from build123d import *

# Parameters (mm, degrees)
F1_DEPTH       = 16
F3_D           = 3.15
F3_CBORE_D     = 6.5
F3_CBORE_DEPTH = 3


with BuildPart() as f1:
    # F0 (on Top) → F1 (new body, symmetric)
    with BuildSketch(Plane.XY):
        with BuildLine():
            Line((4, 3), (-4, 3))
            ThreePointArc((-4, 3), (0, -5), (4, 3))
        make_face()
    extrude(amount=F1_DEPTH, both=True)

    # F3 (through all)
    with Locations(Plane(origin=(0, 3, 0), x_dir=(-1, 0, 0), z_dir=(0, 1, 0))):
        with Locations((0, 8), (0, -8)):
            CounterBoreHole(F3_D / 2, F3_CBORE_D / 2, F3_CBORE_DEPTH)


solid = f1.part
Can you work these out from the model? Positions are in its coordinate system, mm. A direction names the side the tool comes from. Coordinates: 2 decimals unless noted, no trailing zeros. Write each loop counter-clockwise with the first axis right and the second up, starting at its lowest first coordinate (ties: lowest second). Pieces come first, ordered by that corner, then holes. Notation, with made-up numbers: (41.25, 50.5) -> (72.25, 50.5) arc R22 cw to (72.25, 81.5) -> close; hole circle Ø9 at (66.5, 12). An arc over 180 degrees is marked (long way). Write item = value, one per line.
(1) If I drill on probe 1 along Z at (x, y) = (0, -1.45) (3 decimals); probe 2 along Z at (x, y) = (0, 1.55); probe 3 along X at (y, z) = (0.75, -11), over which ranges is the centre line in solid material (lowest first)?
Verdict:
probe_1 = -16 to -9.575, -6.425 to 6.425, 9.575 to 16
probe_2 = -16 to -11.25, -4.75 to 4.75, 11.25 to 16
probe_3 = -4.94 to -1.25, 1.25 to 4.94
(2) For pin 1 (2.5 mm diameter, centred on x = 0, z = -8, fed in from +Y); pin 2 (4 mm diameter, centred on x = 0, z = -8, fed in from +Y); pin 3 (2 mm diameter, centred on y = -2.5, z = -2, fed in from +X), each with a flat end and sliding along its axis, tell me the tip position at first contact or that it passes through.
Verdict:
pin_1 = through
pin_2 = 0
pin_3 = 4.77
(3) On a 3-axis mill with a long thin cutter (end or side, diameter ignored), from which of +Z, -Z, +X, -X, +Y, -Y can I reach the whole of each face in a straight line? I mean faces 1 (the face through (0.423, 1.521, -4.778)), 2 (the face through (1.455, -2.539, 7.397)). Say none if no direction works.
Verdict:
face_1 = +Y
face_2 = +Y, -Y
(4) Imagine slicing it at B-B (x = 0). Please give me the cut outline in (y, z) (3 decimals).
Verdict:
outline = (-5, -16) -> (3, -16) -> (3, -11.25) -> (0, -11.25) -> (0, -9.575) -> (-5, -9.575) -> close; (-5, -6.425) -> (0, -6.425) -> (0, -4.75) -> (3, -4.75) -> (3, 4.75) -> (0, 4.75) -> (0, 6.425) -> (-5, 6.425) -> close; (-5, 9.575) -> (0, 9.575) -> (0, 11.25) -> (3, 11.25) -> (3, 16) -> (-5, 16) -> close
(5) Thinking about a two-plate mould opening in X: for faces 3 (the face through (0, -1, 16)), 4 (the face through (0.423, 1.521, 11.222)), 5 (the face through (0, -5, 0)), which applies, +X half, -X half, draft (parallel to the pull), parting line (faces both ways), or undercut?
Verdict:
face_3 = draft
face_4 = undercut
face_5 = parting line
(6) Imagine slicing it at C-C (y = -2.5). Please give me the cut outline in (x, z) (3 decimals).
Verdict:
outline = (-4.33, -16) -> (4.33, -16) -> (4.33, 16) -> (-4.33, 16) -> close; hole circle Ø3.15 at (0, -8); hole circle Ø3.15 at (0, 8)
(7) Imagine slicing it at D-D (x = -2). Please give me the cut outline in (y, z).
Verdict:
outline = (-4.58, -16) -> (3, -16) -> (3, -10.56) -> (0, -10.56) -> (0, -5.44) -> (3, -5.44) -> (3, 5.44) -> (0, 5.44) -> (0, 10.56) -> (3, 10.56) -> (3, 16) -> (-4.58, 16) -> close
(8) Imagine slicing it at A-A (z = -8.5). Please give me the cut outline in (x, y).
Verdict:
outline = (-4, 3) arc R5 ccw to (-1.49, -4.77) -> (-1.49, 0) -> (-3.21, 0) -> (-3.21, 3) -> close; (1.49, -4.77) arc R5 ccw to (4, 3) -> (3.21, 3) -> (3.21, 0) -> (1.49, 0) -> close
